```python
from build123d import *

# Parameters (mm, degrees)
SKETCH1_W                      = 1409.7
SKETCH1_H                      = 81.75625
BASE_FLANGE1_DEPTH             = 2.052574
EDGE_FLANGE1_STRIP_W           = 14.560296
EDGE_FLANGE1_STRIP_H           = 2.052574
EDGE_FLANGE1_STRIP_CUT_DEPTH   = 1409.7
EDGE_FLANGE1_STRIP_2_W         = 14.560296
EDGE_FLANGE1_STRIP_2_H         = 2.052574
EDGE_FLANGE1_STRIP_CUT_2_DEPTH = 1409.7
EDGE_FLANGE1_DEPTH             = 1409.7
EDGE_FLANGE1_BEND_DEPTH        = 1409.7
F_7_0_201_DIAMETER_HOLE1_D     = 5.1054
F_0_257_DIAMETER_HOLE1_D       = 6.5278
FILLET1_R                      = 3.175
F_1_1_DIAMETER_HOLE1_D         = 25.4


# Sheet-metal steps are written as plain solids
with BuildPart() as part:
    # Sketch1 → Base-Flange1 (new body)
    with BuildSketch(Plane(origin=(0, 0, 0), x_dir=(1, 0, 0), z_dir=(0, 1, 0))):
        with Locations((704.85, 40.878125)):
            Rectangle(SKETCH1_W, SKETCH1_H)
    extrude(amount=-BASE_FLANGE1_DEPTH)

    # Edge-Flange1 strip (across the edge) → Edge-Flange1 strip cut (cut)
    with BuildSketch(Plane(origin=(0, 0, 0), x_dir=(0, 0, -1), z_dir=(1, 0, 0))):
        with Locations((-2.052574, -1.026287)):
            Rectangle(EDGE_FLANGE1_STRIP_W, EDGE_FLANGE1_STRIP_H)
    extrude(amount=EDGE_FLANGE1_STRIP_CUT_DEPTH, mode=Mode.SUBTRACT)

    # Edge-Flange1 strip 2 (across the edge) → Edge-Flange1 strip cut 2 (cut)
    with BuildSketch(Plane(origin=(1409.7, 0, -81.75625), x_dir=(0, 0, 1), z_dir=(-1, 0, 0))):
        with Locations((-2.052574, -1.026287)):
            Rectangle(EDGE_FLANGE1_STRIP_2_W, EDGE_FLANGE1_STRIP_2_H)
    extrude(amount=EDGE_FLANGE1_STRIP_CUT_2_DEPTH, mode=Mode.SUBTRACT)

    # Edge-Flange1 section (across the edge) → Edge-Flange1 (add)
    with BuildSketch(Plane(origin=(0, 0, 0), x_dir=(0, 0, -1), z_dir=(1, 0, 0))):
        with BuildLine():
            Line((0, 3.175), (0, 48.747426))
            Line((0, 48.747426), (2.052574, 48.747426))
            Line((2.052574, 48.747426), (2.052574, 3.175))
            ThreePointArc((2.052574, 3.175), (2.98250997, 0.92993597), (5.227574, 0))
            Line((5.227574, 0), (5.227574, -2.052574))
            ThreePointArc((5.227574, -2.052574), (1.531120975, -0.521453025), (0, 3.175))
        make_face()
    extrude(amount=EDGE_FLANGE1_DEPTH)

    # Edge-Flange1 section 2 (across the edge) → Edge-Flange1 bend (add)
    with BuildSketch(Plane(origin=(1409.7, 0, -81.75625), x_dir=(0, 0, 1), z_dir=(-1, 0, 0))):
        with BuildLine():
            Line((0, 3.175), (0, 48.747426))
            Line((0, 48.747426), (2.052574, 48.747426))
            Line((2.052574, 48.747426), (2.052574, 3.175))
            ThreePointArc((2.052574, 3.175), (2.98250997, 0.92993597), (5.227574, 0))
            Line((5.227574, 0), (5.227574, -2.052574))
            ThreePointArc((5.227574, -2.052574), (1.531120975, -0.521453025), (0, 3.175))
        make_face()
    extrude(amount=EDGE_FLANGE1_BEND_DEPTH)

    # #7 (0.201) Diameter Hole1 (through all)
    with Locations(Plane(origin=(0, -2.052574, 0), x_dir=(-1, 0, 0), z_dir=(0, -1, 0))):
        with Locations((-1384.3, 40.878125), (-1330.325, 40.878125), (-1357.3125, 67.865625), (-1357.3125, 13.890625)):
            Hole(F_7_0_201_DIAMETER_HOLE1_D / 2)

    # F (0.257) Diameter Hole1 (through all)
    with Locations(Plane.XY):
        with Locations((1358.9, 39.222426), (50.8, 39.222426)):
            Hole(F_0_257_DIAMETER_HOLE1_D / 2)

    # Fillet1
    fillet1_edges = [part.edges().sort_by_distance(p)[0] for p in [
        (0, 48.747426, -1.026287),
        (1409.7, 48.747426, -1.026287),
        (1409.7, 48.747426, -80.729963),
        (0, 48.747426, -80.729963),
    ]]
    fillet(fillet1_edges, radius=FILLET1_R)

    # 1 (1) Diameter Hole1 (through all)
    with Locations(Plane(origin=(0, -2.052574, 0), x_dir=(-1, 0, 0), z_dir=(0, -1, 0))):
        with Locations((-1357.3125, 40.878125)):
            Hole(F_1_1_DIAMETER_HOLE1_D / 2)


solid = part.part
```
Geometry check sheet. Reference: the model listing, model coordinates, mm. A direction names the side the tool comes from. Give positions to 0.01 mm unless a question says otherwise; leave off trailing zeros. Write each loop counter-clockwise with the first axis right and the second up, starting at its lowest first coordinate (ties: lowest second). Pieces come first, ordered by that corner, then holes. Notation, with made-up numbers: (-18, 36) -> (-3, 36) arc R10 cw to (-3, 51) -> close; hole circle Ø1 at (8, 38.5). An arc over 180 degrees is marked (long way). Use one line per item in the form item = value.
Item 1: Sectioned sample at A-A on y = 21.5. Enter the section's corners in (x, z).
Results list:
outline = (0, -81.76) -> (1409.7, -81.76) -> (1409.7, -79.7) -> (0, -79.7) -> close; (0, -2.05) -> (1409.7, -2.05) -> (1409.7, 0) -> (0, 0) -> close
Item 2: Scan lines: line 1 (Z direction, x = 1309, y = 34); line 2 (Y direction, x = 50.8, z = -1.3); line 3 (Z direction, x = 1210, y = 2.5). Record each from-to range of solid material in increasing order.
Results list:
line_1 = -81.76 to -79.7, -2.05 to 0
line_2 = -0.27 to 35.96, 42.49 to 48.75
line_3 = -81.71 to -79.63, -2.13 to -0.04
Item 3: Depth check by flat-ended pin: pin 1 Ø6 at (x, z) = (1384.3, -40.88) entering from +Y; pin 2 Ø20.5 at (x, z) = (1357.31, -40.88) entering from -Y; pin 3 Ø7.5 at (x, y) = (50.8, 39.22) entering from +Z. Enter the tip coordinate at first touch or a pass-through.
Results list:
pin_1 = 0
pin_2 = through
pin_3 = 0
Item 4: Access from +Z, -Z, +X, -X, +Y, -Y to the whole of each face (thin tool, end or side, straight path). Record for faces 1 (the flat face through (695, 26, 0)), 2 (the flat face through (695, 0, -41)).
Results list:
face_1 = +Z, +X, -X, +Y, -Y
face_2 = +X, -X, +Y
Item 5: Sectioned sample at B-B on x = 767. Enter the section's corners in (y, z) (3 decimals).
Results list:
outline = (-2.053, -76.529) arc R5.228 ccw to (3.175, -81.756) -> (48.747, -81.756) -> (48.747, -79.704) -> (3.175, -79.704) arc R3.175 cw to (0, -76.529) -> (0, -5.228) arc R3.175 cw to (3.175, -2.053) -> (48.747, -2.053) -> (48.747, 0) -> (3.175, 0) arc R5.228 ccw to (-2.053, -5.228) -> close
Item 6: Mould release check, pull along X, two halves, no side actions. Record for faces 3 (the flat face through (0, -1, -41)), 4 (the flat face through (1409.7, -1, -41)), 5 (the flat face through (715, 26, -81.756)), 6 (the cylindrical face through (1369.426, -1.012, -44.693)): released by +X, released by -X, zero draft, split by the parting line, or undercut.
Results list:
face_3 = released by -X
face_4 = released by +X
face_5 = zero draft
face_6 = undercut
